Could you check a few things on this model? Use its own coordinates, in mm. A direction names the side the tool comes from. Give positions to 0.01 mm unless a question says otherwise; leave off trailing zeros. Write each loop counter-clockwise with the first axis right and the second up, starting at its lowest first coordinate (ties: lowest second). Pieces come first, ordered by that corner, then holes. Notation, with made-up numbers: (18.5, 38) - (66.5, 38) arc R24 cw to (66.5, 62) - close; hole circle Ø8 at (-35, -18). An arc over 180 degrees is marked (long way). Write item = value, one per line.
from build123d import *

# Parameters (mm, degrees)
F0_W     = 50
F0_H     = 50
F1_DEPTH = 500
F2_R     = 6
F3_T     = -3
F4_R     = 17.526
F5_DEPTH = 25


with BuildPart() as f1:
    # F0 (on Front) → F1 (new body)
    with BuildSketch(Plane.XZ):
        Rectangle(F0_W, F0_H)
    extrude(amount=F1_DEPTH)

    # F2
    f2_edges = [f1.edges().sort_by_distance(p)[0] for p in [
        (25, -250, 25),
        (-25, -250, 25),
        (25, -250, -25),
        (-25, -250, -25),
    ]]
    fillet(f2_edges, radius=F2_R)

    # F3
    f3_openings = [f1.faces().sort_by_distance(p)[0] for p in [
        (0, 0, 0),
        (0, -500, 0),
    ]]
    offset(amount=F3_T, openings=f3_openings)

    # F4 (on face) → F5 (join)
    with BuildSketch(Plane.XY.offset(25)):
        with BuildLine():
            ThreePointArc((19, -259.1351367806), (20.5549108974, -254.6846944404), (21.082, -250))
            ThreePointArc((21.082, -250), (20.5549108974, -245.3153055596), (19, -240.8648632194))
            Line((19, -240.8648632194), (19, -259.1351367806))
        make_face()
        with BuildLine():
            Line((19, -259.1351367806), (19, -240.8648632194))
            ThreePointArc((19, -240.8648632194), (0, -228.918), (-19, -240.8648632194))
            Line((-19, -240.8648632194), (-19, -259.1351367806))
            ThreePointArc((-19, -259.1351367806), (0, -271.082), (19, -259.1351367806))
        make_face()
        with Locations((0, -250)):
            Circle(F4_R, mode=Mode.SUBTRACT)
        with BuildLine():
            Line((-19, -259.1351367806), (-19, -240.8648632194))
            ThreePointArc((-19, -240.8648632194), (-21.082, -250), (-19, -259.1351367806))
        make_face()
    extrude(amount=F5_DEPTH)


solid = f1.part
1. For pin 1 (8 mm diameter, centred on x = 2.5, y = -442, fed in from +Z); pin 2 (8 mm diameter, centred on x = 4.5, z = 16.5, fed in from -Y); pin 3 (8 mm diameter, centred on x = -13, z = 31, fed in from +Y); pin 4 (8 mm diameter, centred on x = 12, z = 42, fed in from +Y), each with a flat end and sliding along its axis, tell me the tip position at first contact or that it passes through.
Filled sheet:
pin_1 = 25
pin_2 = through
pin_3 = -230.94
pin_4 = -230.49
2. If we section it at C-C, the plane z = -6.5: Please give me the cut outline in (x, y).
Filled sheet:
outline = (-25, -500) - (-22, -500) - (-22, 0) - (-25, 0) - close; (22, -500) - (25, -500) - (25, 0) - (22, 0) - close
3. I need wall thicknesses on line 1 (Z direction, x = 4.5, y = -369.5); line 2 (Y direction, x = 0, z = 41.25). Which ranges of each line are inside material? Lowest first, please.
Filled sheet:
line_1 = -25 to -22, 22 to 25
line_2 = -271.08 to -267.53, -232.47 to -228.92
4. Which directions (+Z, -Z, +X, -X, +Y, -Y) give clear straight access to the entire face, cutting with the end or side of a thin tool? Please do faces 5 (the face through (-8, -234, 50)), 6 (the face through (22, -246, 0)), 7 (the face through (0, -250, 25)).
Filled sheet:
face_5 = +Z, +X, -X, +Y, -Y
face_6 = +Y, -Y
face_7 = +Z
5. If we section it at A-A, the plane x = 0: Please give me the cut outline in (y, z), and give its area (3 significant figures).
Filled sheet:
outline = (-500, -25) - (0, -25) - (0, -22) - (-500, -22) - close; (-500, 22) - (0, 22) - (0, 25) - (-228.92, 25) - (-228.92, 50) - (-232.47, 50) - (-232.47, 25) - (-267.53, 25) - (-267.53, 50) - (-271.08, 50) - (-271.08, 25) - (-500, 25) - close
area = 3,180 mm2
6. If we section it at D-D, the plane z = 35: Please give me the cut outline in (x, y).
Filled sheet:
outline = circle Ø42.16 at (0, -250); hole circle Ø35.05 at (0, -250)
7. Thinking about a two-plate mould opening in Z: for faces 1 (the face through (0, -119, 25)), 2 (the face through (0, -246, -25)), 3 (the face through (-22.3, -500, 0.1)), 4 (the face through (0, -246, 22)), which applies, pulls with the +Z half, pulls with the -Z half, needs draft (parallel to the pull), parting line crosses it, or undercut?
Filled sheet:
face_1 = pulls with the +Z half
face_2 = pulls with the -Z half
face_3 = needs draft
face_4 = undercut
8. If we section it at B-B, the plane y = -458: Please give me the cut outline in (x, z).
Filled sheet:
outline = (-25, -19) arc R6 ccw to (-19, -25) - (19, -25) arc R6 ccw to (25, -19) - (25, 19) arc R6 ccw to (19, 25) - (-19, 25) arc R6 ccw to (-25, 19) - close; hole (-22, -19) arc R3 ccw to (-19, -22) - (19, -22) arc R3 ccw to (22, -19) - (22, 19) arc R3 ccw to (19, 22) - (-19, 22) arc R3 ccw to (-22, 19) - close
